Job drawing, mm, ordinate dimensions from the low corner. One solid piece. A direction names the side the tool comes from. Give positions to 0.01 mm unless a question says otherwise; leave off trailing zeros. Order: outer loops, then holes, each group sorted by start corner. A loop starts at its lowest first (then second) coordinate and runs counter-clockwise, first axis right, second up. Notation, with made-up numbers: (-34.75, 28.25) - (22.25, 28.25) arc R28 cw to (22.25, 66.25) - close; hole circle Ø3 at (37, 75). An arc over 180 degrees is marked (long way). Use one line per item in the form item = value. Start each with the question number.
1. Drill centre lines: line 1 (Y direction, x = 3, z = 16); line 2 (Y direction, x = 2, z = 12); line 3 (Y direction, x = 5.75, z = 13.5) (1 decimal). Where is each one in solid material? Low to high.
2. Tool access for the marked faces 5, 6 and 7: list every direction of +Z, -Z, +X, -X, +Y, -Y with a clear straight run to the whole face (end or side of a thin tool).
3. Band-saw the part on D-D, the plane z = 22.5. List the corners of the cut face in (x, y).
4. Pin check, flat tips, straight feed: P1, Ø7, axis at y = 25.4, z = 15.875, coming from the -X side; P2, Ø3, axis at x = 3, z = 19, coming from the +Y side; P3, Ø1, axis at x = 2, z = 24, coming from the +Y side; P4, Ø0.6, axis at x = 3.5, z = 7, coming from the -Y side. Stop position of each tip, or through.
5. Band-saw the part on C-C, the plane y = 25.4. List the corners of the cut face in (x, z).
6. Pull direction Z, two halves, no side cores. Call the marked faces 1, 2, 3 and 4: +Z half, -Z half, draft (parallel to the pull), parting line (faces both ways), or undercut.
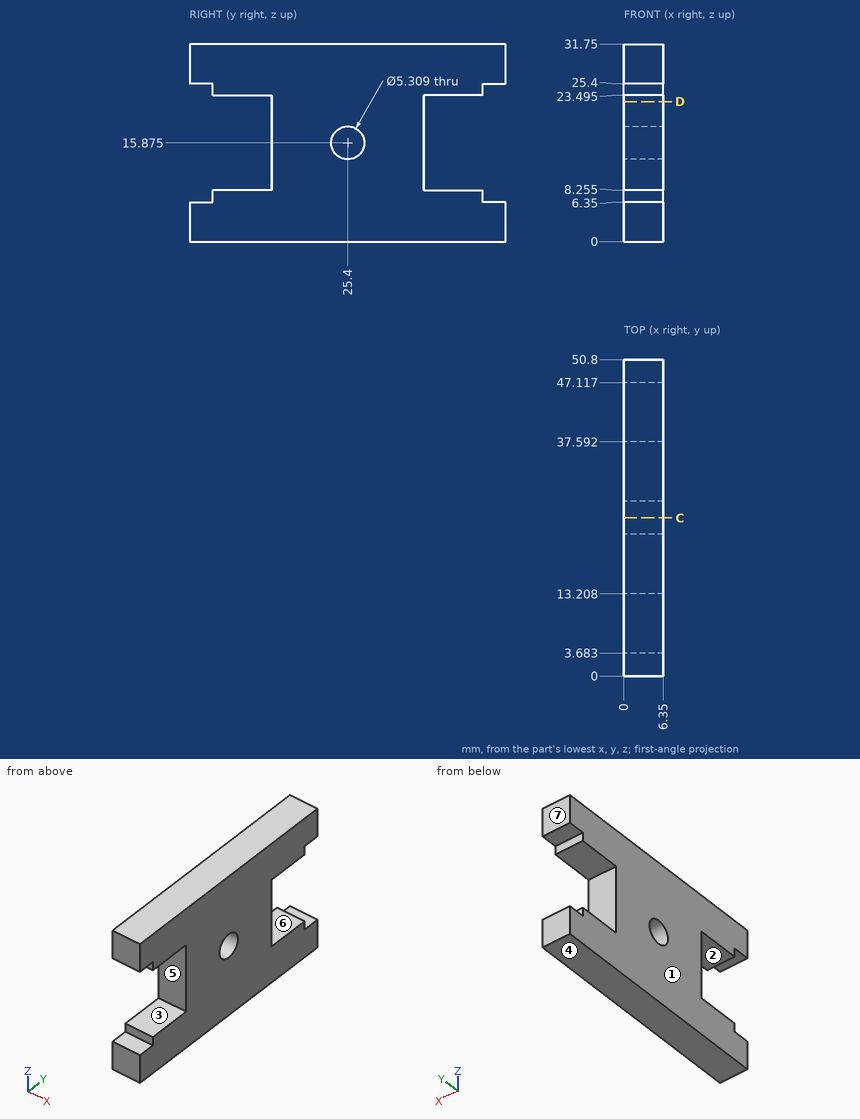
From the geometry:
q1.line_1 = 13.21 to 22.75, 28.05 to 37.59
q1.line_2 = 13.21 to 37.59
q1.line_3 = 13.2 to 24.2, 26.6 to 37.6
q2.face_5 = +X, -X, -Y
q2.face_6 = +X, -X, +Y
q2.face_7 = +Z, -Z, +X, -X, +Y
q3.outline = (0, 13.21) - (6.35, 13.21) - (6.35, 37.59) - (0, 37.59) - close
q4.P1 = 0
q4.P2 = 37.59
q4.P3 = 47.12
q4.P4 = 3.68
q5.outline = (0, 0) - (6.35, 0) - (6.35, 13.22) - (0, 13.22) - close; (0, 18.53) - (6.35, 18.53) - (6.35, 31.75) - (0, 31.75) - close
q6.face_1 = draft
q6.face_2 = undercut
q6.face_3 = undercut
q6.face_4 = -Z half
